CAD build for the part. Positions are in the model's coordinates, mm. A direction names the side the tool comes from. Give positions to 0.01 mm unless a question says otherwise; leave off trailing zeros. Order: outer loops, then holes, each group sorted by start corner. A loop starts at its lowest first (then second) coordinate and runs counter-clockwise, first axis right, second up. Notation, with made-up numbers: (-7, 60.25) -> (0, 60.25) arc R18 ccw to (0, 69.25) -> close; hole circle Ø8 at (26, -26). An arc over 180 degrees is marked (long way). Use one line per item in the form item = value. Start each with the question number.
1) Mould opens along Z. For faces 1 (the face through (3, -3, -6.35)), 2 (the face through (3, 16, 0)), 3 (the face through (3, -3, -19.05)), 4 (the face through (3, 16, -25.4)) say: pulls with the +Z half, pulls with the -Z half, needs draft (parallel to the pull), parting line crosses it, or undercut.
2) Cut at C-C, the plane z = -7. Give the cut face in (x, y).
3) Tool access for faces 5 (the face through (0, 11, -7)), 6 (the face through (3, 0, -13)): list every direction of +Z, -Z, +X, -X, +Y, -Y with a clear straight run to the whole face (end or side of a thin tool).
4) Cut at A-A, the plane x = 5.25. Give the cut face in (y, z), and give its area (3 significant figures).
5) Cut at B-B, the plane y = -3. Give the cut face in (x, z).
6) Probe line 1 (Y direction, x = 3, z = -4.5); line 2 (Z direction, x = 3.25, y = 30); line 3 (Y direction, x = 2.25, z = -4.25). List the from-to ranges inside material, lowest first.
7) Drop a flat-ended pin along its axis: P1, Ø1.9, axis at x = 3.5, z = -12, coming from the -Y side. Give the stop position or say it passes through.
from build123d import *

# Parameters (mm, degrees)
SKETCH1_W           = 6.35
SKETCH1_H           = 6.35
BOSS_EXTRUDE1_DEPTH = 6.35


with BuildPart() as part:
    # Sketch1 → Boss-Extrude1 (new body)
    with BuildSketch(Plane(origin=(0, 0, 0), x_dir=(0, 0, -1), z_dir=(1, 0, 0))):
        with Locations((22.225, -3.175)):
            Rectangle(SKETCH1_W, SKETCH1_H)
        with BuildLine():
            Line((25.4, 38.1), (12.7, 38.1))
            Line((12.7, 38.1), (12.7, 33.02))
            ThreePointArc((12.7, 33.02), (20.782230509, 29.672230509), (24.13, 21.59))
            ThreePointArc((24.13, 21.59), (20.782230509, 13.507769491), (12.7, 10.16))
            Line((12.7, 10.16), (12.7, 0))
            Line((12.7, 0), (19.05, 0))
            Line((19.05, 0), (25.4, 0))
            Line((25.4, 0), (25.4, 38.1))
        make_face()
        with BuildLine():
            Line((12.7, 33.02), (12.7, 38.1))
            Line((12.7, 38.1), (0, 38.1))
            Line((0, 38.1), (0, 0))
            Line((0, 0), (6.35, 0))
            Line((6.35, 0), (12.7, 0))
            Line((12.7, 0), (12.7, 10.16))
            ThreePointArc((12.7, 10.16), (1.27, 21.59), (12.7, 33.02))
        make_face()
        with Locations((3.175, -3.175)):
            Rectangle(SKETCH1_W, SKETCH1_H)
    extrude(amount=BOSS_EXTRUDE1_DEPTH)


solid = part.part
Result:
q1.face_1 = undercut
q1.face_2 = pulls with the +Z half
q1.face_3 = undercut
q1.face_4 = pulls with the -Z half
q2.outline = (0, 0) -> (6.35, 0) -> (6.35, 11.68) -> (0, 11.68) -> close; (0, 31.5) -> (6.35, 31.5) -> (6.35, 38.1) -> (0, 38.1) -> close
q3.face_5 = +Z, -Z, -X, +Y, -Y
q3.face_6 = +X, -X, -Y
q4.outline = (-6.35, -25.4) -> (38.1, -25.4) -> (38.1, 0) -> (-6.35, 0) -> (-6.35, -6.35) -> (0, -6.35) -> (0, -19.05) -> (-6.35, -19.05) -> close; hole circle Ø22.86 at (21.59, -12.7)
q4.area = 638 mm²
q5.outline = (0, -25.4) -> (6.35, -25.4) -> (6.35, -19.05) -> (0, -19.05) -> close; (0, -6.35) -> (6.35, -6.35) -> (6.35, 0) -> (0, 0) -> close
q6.line_1 = -6.35 to 13.63, 29.55 to 38.1
q6.line_2 = -25.4 to -20.44, -4.96 to 0
q6.line_3 = -6.35 to 13.89, 29.29 to 38.1
q7.P1 = 0
